For this review, take the finished solid that the model builds, in its own axes (mm). A direction names the side the tool comes from. Give positions to 0.01 mm unless a question says otherwise; leave off trailing zeros. Write each loop counter-clockwise with the first axis right and the second up, starting at its lowest first coordinate (ties: lowest second). Pieces come first, ordered by that corner, then holes.
1) We need section B-B on z = 8.5. Give the boundary of the cut face in (x, y).
2) Wall thickness on line 1 along X through (y, z) = (-59.75, 1.1); line 2 along X through (y, z) = (69, 4.25); line 3 along X through (y, z) = (-78.5, 3.75): over which ranges is each line inside the solid? List them lowest first.
3) We need section C-C on x = 26. Give the boundary of the cut face in (y, z), and give its area (3 significant figures).
4) Draft analysis for pull direction X (two halves, no side actions). For faces 6 (the face through (9.85, -119, 8)), 7 (the face through (104.658, 32.958, 2.465)), 8 (the face through (119, -9.85, 8)), state which applies: pulls with the +X half, pulls with the -X half, needs draft (parallel to the pull), parting line crosses it, or undercut.
5) Machinability: for faces 1 (the face through (-89.917, 89.406, 2.465)), 2 (the face through (-9.85, 119, 8)), 3 (the face through (0, 109.6, 8)), 4 (the face through (9.85, 119, 8)), 5 (the face through (40.35, 109.82, 2.46)), which of the approach directions +Z, -Z, +X, -X, +Y, -Y give a long, thin tool a straight path to every point of the face, cutting with its end or side? Answer none if there is none.
6) For P1, Ø5, axis at x = -15, y = 119.5, coming from the -Z side; P2, Ø6.5, axis at y = -0.5, z = 7.5, coming from the +X side; P3, Ø6.5, axis at x = 4, z = 8, coming from the -Y side; P4, Ø3, axis at x = -122.5, z = 8, coming from the +Y side, all flat-tipped, find the tip position at first contact; note any pin that passes through.
7) We need section A-A on y = 0. Give the boundary of the cut face in (x, z) (3 decimals), and give its area (3 significant figures).
8) We need section D-D on y = 66. Give the boundary of the cut face in (x, z), and give its area (3 significant figures).
from build123d import *

# Parameters (mm, degrees)
SKETCH2_R           = 129.4
SKETCH2_R_2         = 109.725
SKETCH2_R_3         = 2.75
BOSS_EXTRUDE1_DEPTH = 5
BOSS_EXTRUDE2_DEPTH = 6.1
CUT_EXTRUDE3_DEPTH  = 10
SKETCH5_R           = 2.75
CUT_EXTRUDE4_DEPTH  = 184.335566653


with BuildPart() as part:
    # Sketch2 → Boss-Extrude1 (new body)
    with BuildSketch(Plane.XY):
        Circle(SKETCH2_R)
        Circle(SKETCH2_R_2, mode=Mode.SUBTRACT)
        with Locations(Location((-15, 119.5, 0), (0, 0, 180))):
            Circle(SKETCH2_R_3, mode=Mode.SUBTRACT)
        with Locations((40.94836166, 112.504699024)):
            Circle(SKETCH2_R_3, mode=Mode.SUBTRACT)
        with Locations(Location((119.5, 15, 0), (0, 0, 180))):
            Circle(SKETCH2_R_3, mode=Mode.SUBTRACT)
        with Locations((112.504699024, -40.94836166)):
            Circle(SKETCH2_R_3, mode=Mode.SUBTRACT)
        with Locations(Location((15, -119.5, 0), (0, 0, 180))):
            Circle(SKETCH2_R_3, mode=Mode.SUBTRACT)
        with Locations((-40.94836166, -112.504699024)):
            Circle(SKETCH2_R_3, mode=Mode.SUBTRACT)
        with Locations(Location((-119.5, -15, 0), (0, 0, 180))):
            Circle(SKETCH2_R_3, mode=Mode.SUBTRACT)
        with Locations((-112.504699024, 40.94836166)):
            Circle(SKETCH2_R_3, mode=Mode.SUBTRACT)
    extrude(amount=BOSS_EXTRUDE1_DEPTH)

    # Sketch3 → Boss-Extrude2 (add)
    with BuildSketch(Plane.XY.offset(5)):
        with BuildLine():
            Line((-9.85, 129.024561615), (-9.85, 109.6))
            Line((-9.85, 109.6), (9.85, 109.6))
            Line((9.85, 109.6), (9.85, 129.024561615))
            ThreePointArc((9.85, 129.024561615), (0, 129.4), (-9.85, 129.024561615))
        make_face()
        with BuildLine():
            Line((129.024561615, 9.85), (109.6, 9.85))
            Line((109.6, 9.85), (109.6, -9.85))
            Line((109.6, -9.85), (129.024561615, -9.85))
            ThreePointArc((129.024561615, -9.85), (129.4, 0), (129.024561615, 9.85))
        make_face()
        with BuildLine():
            Line((9.85, -129.024561615), (9.85, -109.6))
            Line((9.85, -109.6), (-9.85, -109.6))
            Line((-9.85, -109.6), (-9.85, -129.024561615))
            ThreePointArc((-9.85, -129.024561615), (0, -129.4), (9.85, -129.024561615))
        make_face()
        with BuildLine():
            Line((-129.024561615, -9.85), (-109.6, -9.85))
            Line((-109.6, -9.85), (-109.6, 9.85))
            Line((-109.6, 9.85), (-129.024561615, 9.85))
            ThreePointArc((-129.024561615, 9.85), (-129.4, 0), (-129.024561615, -9.85))
        make_face()
    extrude(amount=BOSS_EXTRUDE2_DEPTH)

    # Sketch4 → Cut-Extrude3 (cut)
    with BuildSketch(Plane.XY):
        Polygon((126.8, 52.522279709), (52.522279709, 126.8), (53.640656327, 129.5), (129.5, 53.640656327), align=None)
        Polygon((-53.640656327, 129.5), (-129.5, 53.640656327), (-126.8, 52.522279709), (-52.522279709, 126.8), align=None)
        Polygon((-129.5, -53.640656327), (-53.640656327, -129.5), (-52.522279709, -126.8), (-126.8, -52.522279709), align=None)
        Polygon((53.640656327, -129.5), (129.5, -53.640656327), (126.8, -52.522279709), (52.522279709, -126.8), align=None)
    extrude(amount=CUT_EXTRUDE3_DEPTH, mode=Mode.SUBTRACT)

    # Sketch5 → Cut-Extrude4 (cut, through all)
    with BuildSketch(Plane.XY):
        with Locations((103.490035752, 59.75)):
            Circle(SKETCH5_R)
        with Locations((59.75, -103.490035752)):
            Circle(SKETCH5_R)
        with Locations((-103.490035752, -59.75)):
            Circle(SKETCH5_R)
        with Locations((-59.75, 103.490035752)):
            Circle(SKETCH5_R)
    extrude(amount=CUT_EXTRUDE4_DEPTH, mode=Mode.SUBTRACT)


solid = part.part
Results list:
1. outline: (-129.02, -9.85) - (-109.6, -9.85) - (-109.6, 9.85) - (-129.02, 9.85) arc R129.4 ccw to start; (-9.85, -129.02) arc R129.4 ccw to (9.85, -129.02) - (9.85, -109.6) - (-9.85, -109.6) - close; (-9.85, 109.6) - (9.85, 109.6) - (9.85, 129.02) arc R129.4 ccw to (-9.85, 129.02) - close; (109.6, -9.85) - (129.02, -9.85) arc R129.4 ccw to (129.02, 9.85) - (109.6, 9.85) - close
2. line 1: x = -114.78 to -106.24, -100.74 to -92.03, 92.03 to 114.78
2. line 2: x = -109.47 to -85.31, 85.31 to 109.47
2. line 3: x = -100.82 to -76.66, 76.66 to 100.82
3. outline: (-126.76, 0) - (-106.6, 0) - (-106.6, 5) - (-126.76, 5) - close; (106.6, 0) - (126.76, 0) - (126.76, 5) - (106.6, 5) - close
3. area: 202 mm2
4. face 6: pulls with the +X half
4. face 7: undercut
4. face 8: needs draft
5. face 1: +Z, -Z, -X, +Y
5. face 2: +Z, -X, +Y, -Y
5. face 3: +Z, +X, -X
5. face 4: +Z, +X, +Y, -Y
5. face 5: +Z, -Z
6. P1: passes through
6. P2: stops at x = 129.4
6. P3: stops at y = -129.4
6. P4: stops at y = 9.85
7. outline: (-129.4, 0) - (-109.725, 0) - (-109.725, 5) - (-109.6, 5) - (-109.6, 11.1) - (-129.4, 11.1) - close; (109.6, 5) - (109.725, 5) - (109.725, 0) - (129.4, 0) - (129.4, 11.1) - (109.6, 11.1) - close
7. area: 438 mm2
8. outline: (-111.3, 0) - (-87.66, 0) - (-87.66, 5) - (-111.3, 5) - close; (87.66, 0) - (111.3, 0) - (111.3, 5) - (87.66, 5) - close
8. area: 236 mm2
